```python
from build123d import *

# Parameters (mm, degrees)
F1_W         = 50
F1_H         = 17
F1_R         = 1.7
F2_DEPTH     = 6
F4_DEPTH     = 32
F5_T4_ANGLE  = 237.2117204573
F5_T10_ANGLE = 237.2117204573
F6_R         = 6
F7_DEPTH     = 25
F8_R         = 1.5
F9_DEPTH     = 15.2


# Not quite as in the source:
# - a fillet or chamfer that OpenCascade refuses, or shapes differently, is made with other operations: its cross-section is extruded or revolved along the edge and cut away or added


with BuildPart() as f2:
    # F1 (on offset) → F2 (new body)
    with BuildSketch(Plane.XY.offset(70)):
        Rectangle(F1_W, F1_H)
        with Locations((-17, 0)):
            Circle(F1_R, mode=Mode.SUBTRACT)
        with Locations((17, 0)):
            Circle(F1_R, mode=Mode.SUBTRACT)
    extrude(amount=-F2_DEPTH)

    # F3 (on face) → F4 (join)
    with BuildSketch(Plane.XY.offset(70)):
        with BuildLine():
            ThreePointArc((2.9580398915, -8.5), (7.3356103708, -5.2142900272), (9, 0))
            ThreePointArc((9, 0), (7.3356103708, 5.2142900272), (2.9580398915, 8.5))
            Line((2.9580398915, 8.5), (-2.9580398916, 8.5))
            ThreePointArc((-2.9580398916, 8.5), (-9, 0), (-2.9580398916, -8.5))
            Line((-2.9580398916, -8.5), (2.9580398915, -8.5))
        make_face()
        with BuildLine():
            ThreePointArc((-2.9580398916, -8.5), (0, -9), (2.9580398915, -8.5))
            Line((2.9580398915, -8.5), (-2.9580398916, -8.5))
        make_face()
        with BuildLine():
            Line((-2.9580398916, 8.5), (2.9580398915, 8.5))
            ThreePointArc((2.9580398915, 8.5), (0, 9), (-2.9580398916, 8.5))
        make_face()
    extrude(amount=-F4_DEPTH)

    # F5: fillet of radius 3 on 2 edges, made by hand


with BuildPart() as f5_tool2:
    # F5_s3 → F5_t4 (revolve)
    with BuildSketch(Plane(origin=(0, 0, 0), x_dir=(0, 0, 1), z_dir=(-0.8779340101, 0.4787816558, 0))):
        with BuildLine():
            ThreePointArc((61, -9), (63.1213203436, -9.8786796564), (64, -12))
            Line((64, -12), (64, -9))
            Line((64, -9), (61, -9))
        make_face()
    revolve(axis=Axis((0, 0, 64), (0, 0, 1)), revolution_arc=F5_T4_ANGLE)

    split(bisect_by=Plane.XZ.offset(-8.5), keep=Keep.TOP)

    split(bisect_by=Plane.XZ.offset(8.5), keep=Keep.BOTTOM)


with BuildPart() as f2_1:
    add(f2.part)

    # F5_t1: union F5_tool2
    add(f5_tool2.part)


with BuildPart() as f5_tool8:
    # F5_s9 → F5_t10 (revolve)
    with BuildSketch(Plane(origin=(0, 0, 0), x_dir=(0, 0, 1), z_dir=(0.8779340101, -0.4787816558, 0))):
        with BuildLine():
            ThreePointArc((61, -9), (63.1213203436, -9.8786796564), (64, -12))
            Line((64, -12), (64, -9))
            Line((64, -9), (61, -9))
        make_face()
    revolve(axis=Axis((0, 0, 64), (0, 0, 1)), revolution_arc=F5_T10_ANGLE)

    split(bisect_by=Plane.XZ.offset(-8.5), keep=Keep.TOP)

    split(bisect_by=Plane.XZ.offset(8.5), keep=Keep.BOTTOM)


with BuildPart() as f2_2:
    add(f2_1.part)

    # F5_t7: union F5_tool8
    add(f5_tool8.part)

    # F6 (on face) → F7 (cut)
    with BuildSketch(Plane(origin=(0, 0, 38), x_dir=(1, 0, 0), z_dir=(0, 0, -1))):
        Circle(F6_R)
    extrude(amount=-F7_DEPTH, mode=Mode.SUBTRACT)

    # F8 (on Front) → F9 (cut, symmetric)
    with BuildSketch(Plane.XZ):
        with Locations((0, 48)):
            Circle(F8_R)
    extrude(amount=F9_DEPTH, both=True, mode=Mode.SUBTRACT)


solid = f2_2.part
```
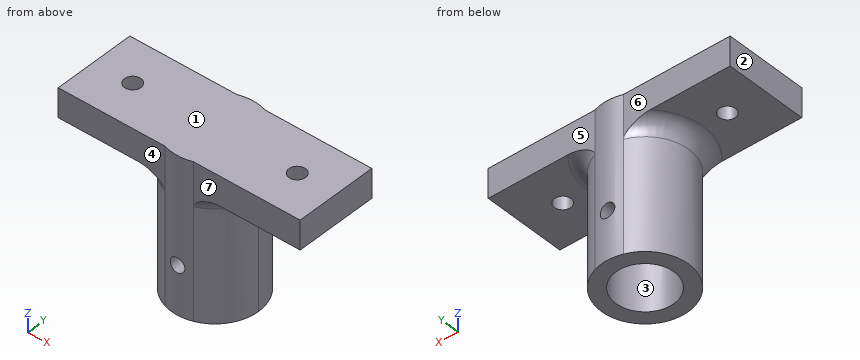
The model under review builds one solid part; all positions refer to its coordinate system, in mm. Face numbers are marked on the shaded views. A direction names the side the tool comes from. Round coordinates to 2 decimals unless told otherwise and drop trailing zeros. Write each loop counter-clockwise with the first axis right and the second up, starting at its lowest first coordinate (ties: lowest second). Pieces come first, ordered by that corner, then holes.
(1) Insertion check: pin 1 (4 mm diameter, centred on y = 1.5, z = 54.5, fed in from +X); pin 2 (8.5 mm diameter, centred on x = 17, y = -1.5, fed in from -Z); pin 3 (10 mm diameter, centred on x = -8.5, z = 64.5, fed in from +Y). Each pin has a flat end and moves straight along its axis. Give the tip position at first contact, or say it passes through.
(2) Machinability: for the marked faces 4, 5, 6 and 7, which of the approach directions +Z, -Z, +X, -X, +Y, -Y give a long, thin tool a straight path to every point of the face, cutting with its end or side? Answer none if there is none.
(3) We need section A-A on x = -17. Give the boundary of the cut face in (y, z), and give its area (3 significant figures).
(4) We need section D-D on z = 48. Give the boundary of the cut face in (x, y), and give its area (3 significant figures).
(5) Wall thickness on L1, parallel to Y at x = -17, z = 67.1; L2, parallel to Z at x = 0, y = 7.5; L3, parallel to Y at x = 0, z = 54.75: over which ranges is each line inside the solid? List them lowest first.
(6) We need section B-B on z = 64.5. Give the boundary of the cut face in (x, y), and give its area (3 significant figures).
(7) Mouldability with a two-part tool opening along X and no side actions: class the marked faces 1, 2 and 3 as +X half, -X half, draft (parallel to the pull), parting line (faces both ways), or undercut.
(8) We need section C-C on x = -0.5. Give the boundary of the cut face in (y, z), and give its area (3 significant figures).
Findings below:
1. pin 1: stops at x = 9
1. pin 2: stops at z = 64
1. pin 3: stops at y = 8.5
2. face 4: +Z, -Z, -X, -Y
2. face 5: +Z, -Z, +X, +Y
2. face 6: +Z, -Z, -X, +Y
2. face 7: +Z, -Z, +X, -Y
3. outline: (-8.5, 64) - (-1.7, 64) - (-1.7, 70) - (-8.5, 70) - close; (1.7, 64) - (8.5, 64) - (8.5, 70) - (1.7, 70) - close
3. area: 81.6 mm2
4. outline: (-1.5, -8.87) - (-1.5, -5.81) arc R6 cw to (-1.5, 5.81) - (-1.5, 8.87) arc R9 ccw to start; (1.5, -8.87) arc R9 ccw to (1.5, 8.87) - (1.5, 5.81) arc R6 cw to (1.5, -5.81) - close
4. area: 123 mm2
5. L1: y = -8.5 to -1.7, 1.7 to 8.5
5. L2: z = 38 to 46.5, 49.5 to 70
5. L3: y = -9 to -6, 6 to 9
6. outline: (-25, -8.5) - (-2.96, -8.5) arc R9 ccw to (2.96, -8.5) - (25, -8.5) - (25, 8.5) - (2.96, 8.5) arc R9 ccw to (-2.96, 8.5) - (-25, 8.5) - close; hole circle Ø3.4 at (-17, 0); hole circle Ø3.4 at (17, 0)
6. area: 836 mm2
7. face 1: draft
7. face 2: -X half
7. face 3: undercut
8. outline: (-8.99, 38) - (-5.98, 38) - (-5.98, 46.59) - (-8.99, 46.59) - close; (-8.99, 49.41) - (-5.98, 49.41) - (-5.98, 63) - (5.98, 63) - (5.98, 49.41) - (8.99, 49.41) - (8.99, 70) - (-8.99, 70) - close; (5.98, 38) - (8.99, 38) - (8.99, 46.59) - (5.98, 46.59) - close
8. area: 259 mm2
